Work out the finished part from the listing and answer in its coordinate system (mm). Give positions to 0.01 mm unless a question says otherwise; leave off trailing zeros. Order: outer loops, then holes, each group sorted by start corner. A loop starts at its lowest first (then second) coordinate and runs counter-clockwise, first axis right, second up.
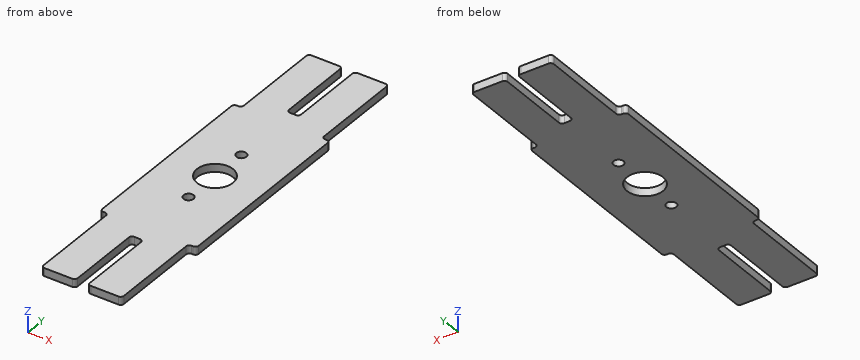
```python
from build123d import *

# Parameters (mm, degrees)
F0_W     = 63.5
F0_H     = 304.8
F1_DEPTH = 6.35
F2_W     = 76.2
F2_H     = 152.4
F3_DEPTH = 6.35
F4_W     = 9.652
F4_H     = 63.5
F4_R     = 14.2875
F4_R_2   = 3.96875
F5_DEPTH = 6.351
F6_R     = 2.54


with BuildPart() as f1:
    # F0 (on Top) → F1 (new body)
    with BuildSketch(Plane.XY):
        Rectangle(F0_W, F0_H)
    extrude(amount=F1_DEPTH)

    # F2 (on Top) → F3 (join)
    with BuildSketch(Plane.XY):
        Rectangle(F2_W, F2_H)
    extrude(amount=F3_DEPTH)

    # F4 (on face) → F5 (cut, through all)
    with BuildSketch(Plane.XY.offset(6.35)):
        with Locations((0, 120.65)):
            Rectangle(F4_W, F4_H)
        with Locations((0, -120.65)):
            Rectangle(F4_W, F4_H)
        Circle(F4_R)
        with Locations((0, 30.1625)):
            Circle(F4_R_2)
        with Locations((0, -30.1625)):
            Circle(F4_R_2)
    extrude(amount=-F5_DEPTH, mode=Mode.SUBTRACT)

    # F6
    f6_edges = [f1.edges().sort_by_distance(p)[0] for p in [
        (-38.1, 76.2, 3.175),
        (-31.75, 76.2, 3.175),
        (-31.75, 152.4, 3.175),
        (-4.826, 152.4, 3.175),
        (4.826, 152.4, 3.175),
        (4.826, 88.9, 3.175),
        (-4.826, 88.9, 3.175),
        (31.75, 152.4, 3.175),
        (31.75, 76.2, 3.175),
        (38.1, 76.2, 3.175),
        (38.1, -76.2, 3.175),
        (31.75, -76.2, 3.175),
        (31.75, -152.4, 3.175),
        (4.826, -152.4, 3.175),
        (4.826, -88.9, 3.175),
        (-4.826, -88.9, 3.175),
        (-4.826, -152.4, 3.175),
        (-31.75, -152.4, 3.175),
        (-31.75, -76.2, 3.175),
        (-38.1, -76.2, 3.175),
    ]]
    fillet(f6_edges, radius=F6_R)


solid = f1.part
```
1. Given P1, Ø3, axis at y = 94.5, z = 3.5, coming from the -X side; P2, Ø2.5, axis at x = -1, z = 1.5, coming from the +Y side; P3, Ø2.5, axis at x = 0.5, z = 2.5, coming from the -Y side, each flat-ended and moving along its own axis, determine where each tip first touches the part or whether it passes through.
Findings below:
P1: stops at x = -31.75
P2: stops at y = 88.9
P3: stops at y = -88.9
2. The part is cut by section B-B (x = -11.5). Write down the section's boundary in (y, z).
Findings below:
outline: (-152.4, 0) - (-8.48, 0) - (-8.48, 6.35) - (-152.4, 6.35) - close; (8.48, 0) - (152.4, 0) - (152.4, 6.35) - (8.48, 6.35) - close
3. The part is cut by section C-C (z = 2). State how many separate pieces and enclosed holes the cut face has, then the cut area to 3 significant figures.
Findings below:
separate pieces: 1
enclosed holes: 3
area: 19,300 mm2
4. Straight lines are drawn through the part: probe 1 along Y at (x, z) = (0, 3.5); probe 2 along X at (y, z) = (132, 1.5); probe 3 along X at (y, z) = (-1, 1.75). For each, find the intervals that lie inside material, in ascending order.
Findings below:
probe 1: y = -88.9 to -34.13, -26.19 to -14.29, 14.29 to 26.19, 34.13 to 88.9
probe 2: x = -31.75 to -4.83, 4.83 to 31.75
probe 3: x = -38.1 to -14.25, 14.25 to 38.1
5. The part is cut by section A-A (y = 96). Write down the section's boundary in (x, z), then the cut area to 3 significant figures.
Findings below:
outline: (-31.75, 0) - (-4.83, 0) - (-4.83, 6.35) - (-31.75, 6.35) - close; (4.83, 0) - (31.75, 0) - (31.75, 6.35) - (4.83, 6.35) - close
area: 342 mm2
